from build123d import *

# Parameters (mm, degrees)
F0_W     = 114.3
F0_H     = 58.674
F1_DEPTH = 57.15
F2_W     = 42.926
F2_H     = 31.75
F3_DEPTH = 143.256
F5_DEPTH = 25.4
F7_DEPTH = 101.092
F8_R     = 12.7
F9_DEPTH = 25.4


with BuildPart() as f1:
    # F0 (on Top) → F1 (new body)
    with BuildSketch(Plane.XY):
        with Locations((7.98354, -3.90625)):
            Rectangle(F0_W, F0_H)
    extrude(amount=F1_DEPTH)

    # F2 (on face) → F3 (cut)
    with BuildSketch(Plane.YZ.offset(65.13354)):
        with Locations((-11.78025, 41.275)):
            Rectangle(F2_W, F2_H)
    extrude(amount=-F3_DEPTH, mode=Mode.SUBTRACT)

    # F4 (on face) → F5 (cut)
    with BuildSketch(Plane.XZ.offset(-9.68275)):
        Polygon((65.13354, 38.1), (65.13354, 57.15), (46.08354, 57.15), align=None)
        Polygon((-49.16646, 38.1), (-30.11646, 57.15), (-49.16646, 57.15), align=None)
    extrude(amount=-F5_DEPTH, mode=Mode.SUBTRACT)

    # F6 (on face) → F7 (cut)
    with BuildSketch(Plane.XZ.offset(33.24325)):
        Polygon((39.73354, 12.7), (-23.76646, 12.7), (-31.098808, 12.7), (-23.76646, 0), (39.73354, 0), (47.065889, 12.7), align=None)
    extrude(amount=-F7_DEPTH, mode=Mode.SUBTRACT)

    # F8 (on face) → F9 (cut)
    with BuildSketch(Plane.XY.offset(25.4)):
        with Locations((7.98354, -11.78025)):
            Circle(F8_R)
    extrude(amount=-F9_DEPTH, mode=Mode.SUBTRACT)


solid = f1.part
Geometry check sheet. Reference: the model listing, model coordinates, mm. A direction names the side the tool comes from. Round coordinates to 2 decimals unless told otherwise and drop trailing zeros. Write each loop counter-clockwise with the first axis right and the second up, starting at its lowest first coordinate (ties: lowest second). Pieces come first, ordered by that corner, then holes. Notation, with made-up numbers: (-19.75, 54.25) -> (25.25, 54.25) arc R16 cw to (25.25, 84.25) -> close; hole circle Ø11 at (62, 54). An arc over 180 degrees is marked (long way). One line per item, written item: value. Start each with the question number.
(1) Access from +Z, -Z, +X, -X, +Y, -Y to the whole of each face (thin tool, end or side, straight path). Record for faces 1 (the flat face through (43.35, -4.32, 6.26)), 2 (the flat face through (65.134, -4, 15)), 3 (the flat face through (9, 9.683, 41)).
(2) Cross-section at A-A, the plane z = 10. Record the cut outline in (x, y), and give its area (3 significant figures).
(3) Draft check along X on faces 4 (the cylindrical face through (5.23, -24.18, 19.14)), 5 (the flat face through (-49.166, -4, 15)), 6 (the flat face through (7, -33.243, 15)). Enter one of: +X half, -X half, draft (parallel to the pull), parting line (faces both ways), or undercut.
(4) Cross-section at B-B, the plane x = 43.5. Record the cut outline in (y, z), and give its area (3 significant figures).
(5) Cross-section at C-C, the plane y = -27. Record the cut outline in (x, z), and give its area (3 significant figures).
(6) Go/stop test with flat-tipped pins: pin 1 Ø21.5 at (x, y) = (-5.5, -9.5) entering from +Z; pin 2 Ø17.5 at (x, y) = (16.5, 2.5) entering from -Z; pin 3 Ø1.5 at (x, z) = (-23.5, 47) entering from -Y; pin 4 Ø3 at (x, z) = (-2.5, 11.5) entering from -Y. Record where each tip stops, or that it passes through.
(7) Scan lines: line 1 (Z direction, x = -12, y = -26.5); line 2 (Z direction, x = 40, y = -21.5); line 3 (Z direction, x = -27, y = -12.5). Record each from-to range of solid material in increasing order. Write a range as [from, to].
(8) Cross-section at D-D, the plane y = -7. Record the cut outline in (x, z).
Answer:
1. face 1: +Y, -Y
1. face 2: +Z, -Z, +X, +Y, -Y
1. face 3: +Z, +X, -X, -Y
2. outline: (-49.17, -33.24) -> (-29.54, -33.24) -> (-29.54, 25.43) -> (-49.17, 25.43) -> close; (45.51, -33.24) -> (65.13, -33.24) -> (65.13, 25.43) -> (45.51, 25.43) -> close
2. area: 2,300 mm²
3. face 4: undercut
3. face 5: -X half
3. face 6: draft
4. outline: (-33.24, 0) -> (25.43, 0) -> (25.43, 6.52) -> (-33.24, 6.52) -> close; (-33.24, 12.7) -> (25.43, 12.7) -> (25.43, 57.15) -> (9.68, 57.15) -> (9.68, 25.4) -> (-33.24, 25.4) -> close
4. area: 1,630 mm²
5. outline: (-49.17, 0) -> (-23.77, 0) -> (-31.1, 12.7) -> (47.07, 12.7) -> (39.73, 0) -> (65.13, 0) -> (65.13, 25.4) -> (-49.17, 25.4) -> close
5. area: 2,000 mm²
6. pin 1: z = 25.4
6. pin 2: z = 12.7
6. pin 3: y = 9.68
6. pin 4: y = -33.24
7. line 1: [12.7, 25.4]
7. line 2: [0, 0.46], [12.7, 25.4]
7. line 3: [0, 5.6], [12.7, 25.4]
8. outline: (-49.17, 0) -> (-23.77, 0) -> (-31.1, 12.7) -> (-3.78, 12.7) -> (-3.78, 25.4) -> (-49.17, 25.4) -> close; (19.75, 12.7) -> (47.07, 12.7) -> (39.73, 0) -> (65.13, 0) -> (65.13, 25.4) -> (19.75, 25.4) -> close
